Geometry check sheet. Reference: the model listing, model coordinates, mm. Face numbers are marked on the shaded views. A direction names the side the tool comes from. Round coordinates to 2 decimals unless told otherwise and drop trailing zeros. Order: outer loops, then holes, each group sorted by start corner. A loop starts at its lowest first (then second) coordinate and runs counter-clockwise, first axis right, second up. Notation, with made-up numbers: (12.25, 53) - (46.25, 53) arc R12 cw to (46.25, 63) - close; hole circle Ø1 at (87.25, 19). An arc over 180 degrees is marked (long way). One line per question, with ' | ' between items. Start each with the question number.
Q1. Sectioned sample at A-A, the plane z = 116. Enter the section's corners in (x, y).
Q2. Gauge pin test, flat end, axial feed: P1, Ø12, axis at x = -1.5, y = 25, coming from the +Z side. Record the tip position at first contact, or that the pin passes through.
Q3. Tool access check on the marked faces 4, 5 and 6. Record the directions out of +Z, -Z, +X, -X, +Y, -Y that give a thin tool (end or side, any length) a straight path to the whole face; none if there is none.
Q4. Mould release check, pull along X, two halves, no side actions. Record for the marked faces 1, 2 and 3: +X half, -X half, draft (parallel to the pull), parting line (faces both ways), or undercut.
Q5. Sectioned sample at B-B, the plane x = -2. Enter the section's corners in (y, z), then the cut area to 3 significant figures.
Q6. Material ranges on line 1 along X through (y, z) = (13, 81); line 2 along Z through (x, y) = (-24, 26), recorded low to high.
```python
from build123d import *

# Parameters (mm, degrees)
BOSS_EXTRUDE1_DEPTH = 40
CUT_EXTRUDE1_REACH  = 259.317
SKETCH2_R           = 1.6
CUT_EXTRUDE2_REACH  = 241.402
SKETCH3_R           = 1.25
LPATTERN1_COUNT     = 6
LPATTERN1_PITCH     = 6.25
CHAMFER1_SIZE       = 10


with BuildPart() as part:
    # Sketch1 → Boss-Extrude1 (new body)
    with BuildSketch(Plane(origin=(0, 0, 0), x_dir=(1, 0, 0), z_dir=(0, 1, 0))):
        Polygon((-45, -230), (-53.038475773, -200), (-53.038475773, 0), (53.038475773, 0), (53.038475773, -200), (45, -230), (42.5, -230), (50.538475773, -200), (50.538475773, -2.5), (-50.538475773, -2.5), (-50.538475773, -200), (-42.5, -230), align=None)
    extrude(amount=BOSS_EXTRUDE1_DEPTH)

    # Sketch2 → Cut-Extrude1 (cut, up to next)
    with BuildSketch(Plane(origin=(-99.485571585, 0, 26.657078565), x_dir=(0.2588190451025251, 0, 0.9659258262890672), z_dir=(-0.9659258262890671, 0, 0.25881904510252507)), mode=Mode.PRIVATE) as cut_extrude1_sk1:
        with Locations((186.157797605, 32)):
            Circle(SKETCH2_R)
    cut_extrude1_tool1 = extrude(cut_extrude1_sk1.sketch, amount=-CUT_EXTRUDE1_REACH, mode=Mode.PRIVATE) & part.part
    # Sketch2 → Cut-Extrude1 (cut, up to next)
    with BuildSketch(Plane(origin=(-99.485571585, 0, 26.657078565), x_dir=(0.2588190451025251, 0, 0.9659258262890672), z_dir=(-0.9659258262890671, 0, 0.25881904510252507)), mode=Mode.PRIVATE) as cut_extrude1_sk2:
        with Locations((186.157797605, 8)):
            Circle(SKETCH2_R)
    cut_extrude1_tool2 = extrude(cut_extrude1_sk2.sketch, amount=-CUT_EXTRUDE1_REACH, mode=Mode.PRIVATE) & part.part
    # Sketch2 → Cut-Extrude1 (cut, up to next)
    with BuildSketch(Plane(origin=(-99.485571585, 0, 26.657078565), x_dir=(0.2588190451025251, 0, 0.9659258262890672), z_dir=(-0.9659258262890671, 0, 0.25881904510252507)), mode=Mode.PRIVATE) as cut_extrude1_sk3:
        with Locations((203.157797605, 8)):
            Circle(SKETCH2_R)
    cut_extrude1_tool3 = extrude(cut_extrude1_sk3.sketch, amount=-CUT_EXTRUDE1_REACH, mode=Mode.PRIVATE) & part.part
    # Sketch2 → Cut-Extrude1 (cut, up to next)
    with BuildSketch(Plane(origin=(-99.485571585, 0, 26.657078565), x_dir=(0.2588190451025251, 0, 0.9659258262890672), z_dir=(-0.9659258262890671, 0, 0.25881904510252507)), mode=Mode.PRIVATE) as cut_extrude1_sk4:
        with Locations((203.157797605, 32)):
            Circle(SKETCH2_R)
    cut_extrude1_tool4 = extrude(cut_extrude1_sk4.sketch, amount=-CUT_EXTRUDE1_REACH, mode=Mode.PRIVATE) & part.part
    # Sketch2 → Cut-Extrude1 (cut, up to next)
    with BuildSketch(Plane(origin=(-99.485571585, 0, 26.657078565), x_dir=(0.2588190451025251, 0, 0.9659258262890672), z_dir=(-0.9659258262890671, 0, 0.25881904510252507)), mode=Mode.PRIVATE) as cut_extrude1_sk5:
        with Locations((203.157797605, 20)):
            Circle(SKETCH2_R)
    cut_extrude1_tool5 = extrude(cut_extrude1_sk5.sketch, amount=-CUT_EXTRUDE1_REACH, mode=Mode.PRIVATE) & part.part
    # Sketch2 → Cut-Extrude1 (cut, up to next)
    with BuildSketch(Plane(origin=(-99.485571585, 0, 26.657078565), x_dir=(0.2588190451025251, 0, 0.9659258262890672), z_dir=(-0.9659258262890671, 0, 0.25881904510252507)), mode=Mode.PRIVATE) as cut_extrude1_sk6:
        with Locations((186.157797605, 20)):
            Circle(SKETCH2_R)
    cut_extrude1_tool6 = extrude(cut_extrude1_sk6.sketch, amount=-CUT_EXTRUDE1_REACH, mode=Mode.PRIVATE) & part.part
    cut_extrude1_1 = cut_extrude1_tool1.solids().sort_by_distance((-51.304388, 32, 206.471703))[0]
    add(cut_extrude1_1, mode=Mode.SUBTRACT)
    cut_extrude1_2 = cut_extrude1_tool2.solids().sort_by_distance((-51.304388, 8, 206.471703))[0]
    add(cut_extrude1_2, mode=Mode.SUBTRACT)
    cut_extrude1_3 = cut_extrude1_tool3.solids().sort_by_distance((-46.904464, 8, 222.892442))[0]
    add(cut_extrude1_3, mode=Mode.SUBTRACT)
    cut_extrude1_4 = cut_extrude1_tool4.solids().sort_by_distance((-46.904464, 32, 222.892442))[0]
    add(cut_extrude1_4, mode=Mode.SUBTRACT)
    cut_extrude1_5 = cut_extrude1_tool5.solids().sort_by_distance((-46.904464, 20, 222.892442))[0]
    add(cut_extrude1_5, mode=Mode.SUBTRACT)
    cut_extrude1_6 = cut_extrude1_tool6.solids().sort_by_distance((-51.304388, 20, 206.471703))[0]
    add(cut_extrude1_6, mode=Mode.SUBTRACT)
    cut_extrude1 = cut_extrude1_1 + cut_extrude1_2 + cut_extrude1_3 + cut_extrude1_4 + cut_extrude1_5 + cut_extrude1_6  # Cut-Extrude1 as one shape, for the pattern or mirror that repeats it

    # Mirror1: Cut-Extrude1 across plane
    add(cut_extrude1.mirror(Plane(origin=(0, 0, 0), x_dir=(0, 0, 1), z_dir=(1, 0, 0))), mode=Mode.SUBTRACT)

    # Sketch3 → Cut-Extrude2 (cut, up to next)
    with BuildSketch(Plane(origin=(0, 0, 0), x_dir=(-1, 0, 0), z_dir=(0, 0, -1)), mode=Mode.PRIVATE) as cut_extrude2_sk1:
        with Locations((-10.5, 35)):
            Circle(SKETCH3_R)
    cut_extrude2_tool1 = extrude(cut_extrude2_sk1.sketch, amount=-CUT_EXTRUDE2_REACH, mode=Mode.PRIVATE) & part.part
    # Sketch3 → Cut-Extrude2 (cut, up to next)
    with BuildSketch(Plane(origin=(0, 0, 0), x_dir=(-1, 0, 0), z_dir=(0, 0, -1)), mode=Mode.PRIVATE) as cut_extrude2_sk2:
        with Locations((10.5, 35)):
            Circle(SKETCH3_R)
    cut_extrude2_tool2 = extrude(cut_extrude2_sk2.sketch, amount=-CUT_EXTRUDE2_REACH, mode=Mode.PRIVATE) & part.part
    cut_extrude2_1 = cut_extrude2_tool1.solids().sort_by_distance((10.5, 35, 0))[0]
    add(cut_extrude2_1, mode=Mode.SUBTRACT)
    cut_extrude2_2 = cut_extrude2_tool2.solids().sort_by_distance((-10.5, 35, 0))[0]
    add(cut_extrude2_2, mode=Mode.SUBTRACT)
    cut_extrude2 = cut_extrude2_1 + cut_extrude2_2  # Cut-Extrude2 as one shape, for the pattern or mirror that repeats it

    # LPattern1: Cut-Extrude2 ×6
    with Locations(*[(0, -i * LPATTERN1_PITCH, 0) for i in range(1, LPATTERN1_COUNT)]):
        add(cut_extrude2, mode=Mode.SUBTRACT)

    # Chamfer1
    chamfer1_edges = [part.edges().sort_by_distance(p)[0] for p in [
        (-53.038475773, 20, 0),
        (53.038475773, 20, 0),
        (50.538475773, 20, 2.5),
        (-50.538475773, 20, 2.5),
    ]]
    chamfer(chamfer1_edges, length=CHAMFER1_SIZE)


solid = part.part
```
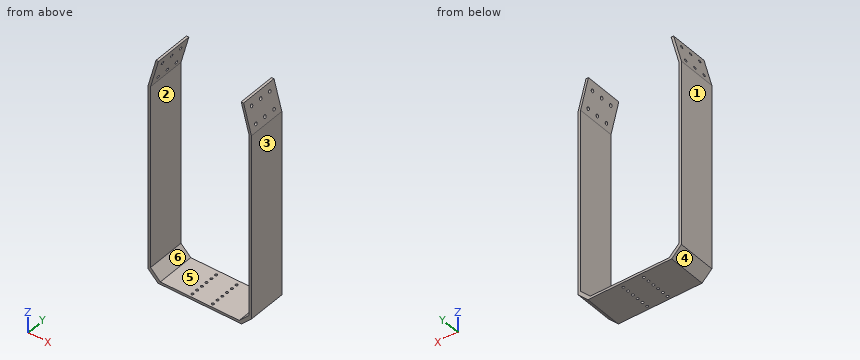
Determined:
1) outline: (-53.04, 0) - (-50.54, 0) - (-50.54, 40) - (-53.04, 40) - close; (50.54, 0) - (53.04, 0) - (53.04, 40) - (50.54, 40) - close
2) P1: stops at z = 2.5
3) face 4: -Z, -X, +Y, -Y | face 5: +Z, +Y, -Y | face 6: +Y, -Y
4) face 1: -X half | face 2: undercut | face 3: +X half
5) outline: (0, 0) - (40, 0) - (40, 2.5) - (0, 2.5) - close | area: 100 mm2
6) line 1: x = -53.04 to -50.54, 50.54 to 53.04 | line 2: z = 0 to 2.5
